Design review of the part shown in the three views and the two pictorial views. Dimensions are in mm from the part's minimum x, y and z. Round coordinates to 2 decimals unless told otherwise and drop trailing zeros. Loops run counter-clockwise (first coordinate to the right, second up) from the corner with the lowest first, then second, coordinate; pieces in that order, holes last.
1) Take a section at C-C (z = 17). State the section outline as (x, y) points.
2) Take a section at D-D (z = 4). State the section outline as (x, y) points, then the cut area to 3 significant figures.
3) Wall thickness on L1, parallel to Y at x = 5, z = 17.5; L2, parallel to Z at x = 3.25, y = 4.75; L3, parallel to X at y = 4.25, z = 15: over which ranges is each line inside the solid? List them lowest first.
4) Insertion check: pin 1 (1.5 mm diameter, centred on y = 1, z = 11.5, fed in from +X); pin 2 (1 mm diameter, centred on x = 6.5, z = 12, fed in from +Y); pin 3 (1.8 mm diameter, centred on x = 6.5, y = 4, fed in from +Z). Each pin has a flat end and moves straight along its axis. Give the tip position at first contact, or say it passes through.
5) Take a section at A-A (y = 5). State the section outline as (x, z) points, then the cut area to 3 significant figures.
6) Mouldability with a two-part tool opening along X and no side actions: class the marked faces 1, 2 and 3 as pulls with the +X half, pulls with the -X half, needs draft (parallel to the pull), parting line crosses it, or undercut.
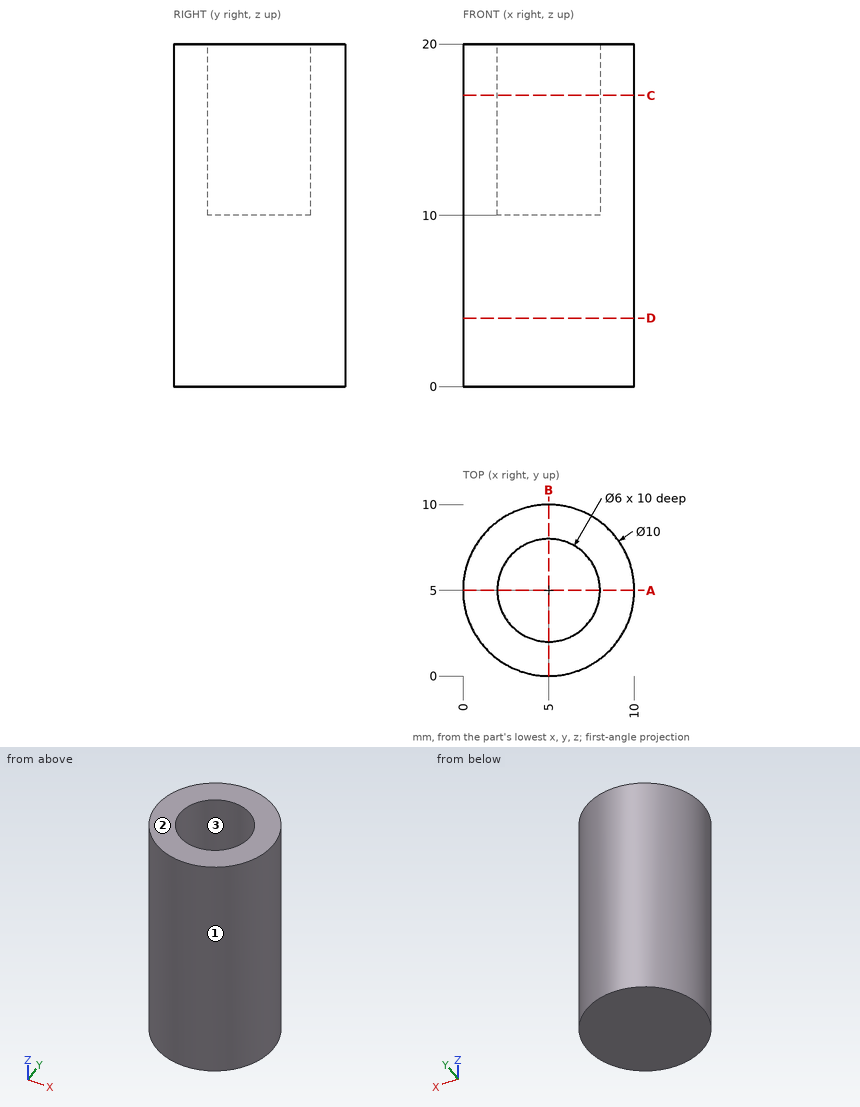
Response:
1. outline: circle Ø10 at (5, 5); hole circle Ø6 at (5, 5)
2. outline: circle Ø10 at (5, 5)
2. area: 78.5 mm2
3. L1: y = 0 to 2, 8 to 10
3. L2: z = 0 to 10
3. L3: x = 0.06 to 2.1, 7.9 to 9.94
4. pin 1: stops at x = 8.8
4. pin 2: stops at y = 9.9
4. pin 3: stops at z = 10
5. outline: (0, 0) - (10, 0) - (10, 20) - (8, 20) - (8, 10) - (2, 10) - (2, 20) - (0, 20) - close
5. area: 140 mm2
6. face 1: parting line crosses it
6. face 2: needs draft
6. face 3: undercut
